```python
from build123d import *

# Parameters (mm, degrees)
SKETCH1_R           = 1.75
BOSS_EXTRUDE1_DEPTH = 1.25
SKETCH2_R           = 10
BOSS_EXTRUDE2_DEPTH = 9.5
FILLET1_R           = 10


with BuildPart() as part:
    # Sketch1 → Boss-Extrude1 (new, symmetric)
    with BuildSketch(Plane(origin=(0, 0, 0), x_dir=(1, 0, 0), z_dir=(0, 1, 0))):
        with BuildLine():
            Line((-14.5, -14), (14.5, -14))
            ThreePointArc((14.5, -14), (20.156854249, -11.656854249), (22.5, -6))
            Line((22.5, -6), (22.5, 6))
            ThreePointArc((22.5, 6), (20.156854249, 11.656854249), (14.5, 14))
            Line((14.5, 14), (-14.5, 14))
            ThreePointArc((-14.5, 14), (-20.156854249, 11.656854249), (-22.5, 6))
            Line((-22.5, 6), (-22.5, -6))
            ThreePointArc((-22.5, -6), (-20.156854249, -11.656854249), (-14.5, -14))
        make_face()
        with Locations(Location((16.5, 0, 0), (0, 0, 270))):
            Circle(SKETCH1_R, mode=Mode.SUBTRACT)
        with Locations(Location((-16.5, 0, 0), (0, 0, 270))):
            Circle(SKETCH1_R, mode=Mode.SUBTRACT)
    extrude(amount=BOSS_EXTRUDE1_DEPTH, both=True)

    # Sketch2 → Boss-Extrude2 (add)
    with BuildSketch(Plane(origin=(0, 1.25, 0), x_dir=(1, 0, 0), z_dir=(0, 1, 0))):
        with Locations(Location((0, 0, 0), (0, 0, 270))):
            Circle(SKETCH2_R)
    extrude(amount=BOSS_EXTRUDE2_DEPTH)

    # Fillet1
    # the kernel refuses this fillet: 10 mm, written as the material it takes off along each edge
    with BuildSketch(Plane(origin=(0, 10.75, 0), x_dir=(0, 0, 1), z_dir=(-1, 0, 0))) as fillet1_piece_1:
        with BuildLine():
            CenterArc((0.012507822, -10), FILLET1_R, 2.865983983, 87.134016017)
            Line((0.012507822, 0), (0.012507822, 0.2))
            Line((0.012507822, 0.2), (10, 0.2))
            Line((10, 0.2), (10.2, 0))
            ThreePointArc((10.2, 0), (10.2, -4.75), (10.199749844, -9.49))
            Line((10.199749844, -9.49), (10, -9.5))
        make_face()
    revolve(axis=Axis((0, 10.75, 0), (0, 1, 0)), mode=Mode.SUBTRACT)


solid = part.part
```
Verification items for the finished model (mm, model axes). A direction names the side the tool comes from. Give positions to 0.01 mm unless a question says otherwise; leave off trailing zeros. Loops run counter-clockwise (first coordinate to the right, second up) from the corner with the lowest first, then second, coordinate; pieces in that order, holes last. Notation, with made-up numbers: M 60.25,80 L 114.25,80 A19 cw 114.25,100 Z; hole C -36,54.5 d9. An arc over 180 degrees is marked long. Return JSON: item names as keys, results as strings.
1) Gauge pin test, flat end, axial feed: P1, Ø4.5, axis at x = -16.5, z = 0, coming from the +Y side. Record the tip position at first contact, or that the pin passes through.
Findings:
{"P1": "stops at y = 1.25"}
2) Section check A-A, the plane x = 16.5. Enter the section's corners in (y, z), and give its area (3 significant figures).
Findings:
{"outline": "M -1.25,-13.75 L 1.25,-13.75 L 1.25,-1.75 L -1.25,-1.75 Z; M -1.25,1.75 L 1.25,1.75 L 1.25,13.75 L -1.25,13.75 Z", "area": "60.0 mm2"}
3) Mould release check, pull along Z, two halves, no side actions. Record for faces 3 (the flat face through (0, 0, 14)), 4 (the cylindrical face through (18.235, -0.018, -0.228)), 5 (the flat face through (22.5, 0, 0)): released by +Z, released by -Z, zero draft, split by the parting line, or undercut.
Findings:
{"face 3": "released by +Z", "face 4": "undercut", "face 5": "zero draft"}
4) Section check B-B, the plane x = -12. Enter the section's corners in (y, z).
Findings:
{"outline": "M -1.25,-14 L 1.25,-14 L 1.25,14 L -1.25,14 Z"}
5) Tool access check on faces 1 (the flat face through (-10.3, 1.25, -0.2)), 2 (the cylindrical face through (-20.219, 0.018, 11.594)). Record the directions out of +Z, -Z, +X, -X, +Y, -Y that give a thin tool (end or side, any length) a straight path to the whole face; none if there is none.
Findings:
{"face 1": "+Y", "face 2": "+Z, -X, +Y, -Y"}
6) Material ranges on L1, parallel to X at y = 0.7, z = 0; L2, parallel to Y at x = 16, z = 4; L3, parallel to Z at x = 15, y = 0.5, recorded low to high. Write a range as [from, to].
Findings:
{"L1": "x = [-22.5, -18.25], [-14.75, 14.75], [18.25, 22.5]", "L2": "y = [-1.25, 1.25]", "L3": "z = [-13.98, -0.9], [0.9, 13.98]"}
7) Section check C-C, the plane z = -11.5. Enter the section's corners in (x, y), and give its area (3 significant figures).
Findings:
{"outline": "M -20.31,-1.25 L 20.31,-1.25 L 20.31,1.25 L -20.31,1.25 Z", "area": "102 mm2"}
